from build123d import *

# Parameters (mm, degrees)
F0_R     = 2
F0_R_2   = 3
F0_R_3   = 1.5
F0_R_4   = 5
F1_DEPTH = 5
F2_R     = 1
F3_R     = 5
F4_DEPTH = 7
F6_W     = 20.916191861
F6_H     = 23.5347189009
F6_W_2   = 37.2305270284
F6_H_2   = 26.8968194723
F7_DEPTH = 25
F8_R     = 5


# Not quite as in the source:
# - a fillet or chamfer that OpenCascade refuses, or shapes differently, is made with other operations: its cross-section is extruded or revolved along the edge and cut away or added


with BuildPart() as f1:
    # F0 (on Top) → F1 (new body)
    with BuildSketch(Plane.XY):
        Polygon((-49.7560231508, 7), (-49.7560231508, 0), (76.2439768492, 0), (76.2439768492, 7), (33.2439768492, 7), (-6.7560231508, 7), align=None)
        with Locations((-45.7560231508, 3)):
            Circle(F0_R, mode=Mode.SUBTRACT)
        with Locations((72.2439768492, 3)):
            Circle(F0_R, mode=Mode.SUBTRACT)
        Polygon((-49.7560231508, 93.5), (-49.7560231508, 7), (-6.7560231508, 7), (-6.7560231508, 12), (33.2439768492, 12), (33.2439768492, 7), (76.2439768492, 7), (76.2439768492, 93.5), (33.2439768492, 93.5), (33.2439768492, 88.5), (-6.7560231508, 88.5), (-6.7560231508, 93.5), align=None)
        with Locations((-34.7560231508, 26.25)):
            Circle(F0_R_2, mode=Mode.SUBTRACT)
        with Locations((3.2439768492, 40.25)):
            Circle(F0_R_3, mode=Mode.SUBTRACT)
        with Locations((23.2439768492, 40.25)):
            Circle(F0_R_3, mode=Mode.SUBTRACT)
        with Locations((48.2439768492, 26.25)):
            Circle(F0_R_2, mode=Mode.SUBTRACT)
        with Locations((3.2439768492, 60.25)):
            Circle(F0_R_3, mode=Mode.SUBTRACT)
        with Locations((-34.7560231508, 74.25)):
            Circle(F0_R_2, mode=Mode.SUBTRACT)
        with Locations((13.2439768492, 50.25)):
            Circle(F0_R_4, mode=Mode.SUBTRACT)
        with Locations((23.2439768492, 60.25)):
            Circle(F0_R_3, mode=Mode.SUBTRACT)
        with Locations((48.2439768492, 74.25)):
            Circle(F0_R_2, mode=Mode.SUBTRACT)
        Polygon((-49.7560231508, 98.5), (-49.7560231508, 93.5), (-6.7560231508, 93.5), (33.2439768492, 93.5), (76.2439768492, 93.5), (76.2439768492, 98.5), align=None)
        with Locations((-34.7560231508, 26.25)):
            Circle(F0_R_2)
        with Locations((-34.7560231508, 26.25)):
            Circle(F0_R_3, mode=Mode.SUBTRACT)
        with Locations((-34.7560231508, 74.25)):
            Circle(F0_R_2)
        with Locations((-34.7560231508, 74.25)):
            Circle(F0_R_3, mode=Mode.SUBTRACT)
        with Locations((48.2439768492, 26.25)):
            Circle(F0_R_2)
        with Locations((48.2439768492, 26.25)):
            Circle(F0_R_3, mode=Mode.SUBTRACT)
        with Locations((48.2439768492, 74.25)):
            Circle(F0_R_2)
        with Locations((48.2439768492, 74.25)):
            Circle(F0_R_3, mode=Mode.SUBTRACT)
        with Locations((13.2439768492, 50.25)):
            Circle(F0_R_4)
        with Locations((3.2439768492, 60.25)):
            Circle(F0_R_3)
        with Locations((3.2439768492, 40.25)):
            Circle(F0_R_3)
        with Locations((23.2439768492, 40.25)):
            Circle(F0_R_3)
        with Locations((23.2439768492, 60.25)):
            Circle(F0_R_3)
    extrude(amount=F1_DEPTH)

    # F2
    f2_edges = [f1.edges().sort_by_distance(p)[0] for p in [
        (-6.756023, 12, 2.5),
        (33.243977, 12, 2.5),
        (-6.756023, 7, 2.5),
        (33.243977, 7, 2.5),
        (-6.756023, 88.5, 2.5),
        (-6.756023, 93.5, 2.5),
        (33.243977, 93.5, 2.5),
        (33.243977, 88.5, 2.5),
    ]]
    fillet(f2_edges, radius=F2_R)

    # F3
    f3_edges = [f1.edges().sort_by_distance(p)[0] for p in [
        (-49.756023, 0, 2.5),
        (76.243977, 0, 2.5),
        (76.243977, 98.5, 2.5),
        (-49.756023, 98.5, 2.5),
    ]]
    fillet(f3_edges, radius=F3_R)

    # F0 (on Top) → F4 (join)
    with BuildSketch(Plane.XY):
        with Locations((-34.7560231508, 74.25)):
            Circle(F0_R_2)
        with Locations((-34.7560231508, 74.25)):
            Circle(F0_R_3, mode=Mode.SUBTRACT)
        with Locations((-34.7560231508, 26.25)):
            Circle(F0_R_2)
        with Locations((-34.7560231508, 26.25)):
            Circle(F0_R_3, mode=Mode.SUBTRACT)
        with Locations((48.2439768492, 74.25)):
            Circle(F0_R_2)
        with Locations((48.2439768492, 74.25)):
            Circle(F0_R_3, mode=Mode.SUBTRACT)
        with Locations((48.2439768492, 26.25)):
            Circle(F0_R_2)
        with Locations((48.2439768492, 26.25)):
            Circle(F0_R_3, mode=Mode.SUBTRACT)
    extrude(amount=F4_DEPTH)

    # F5: fillet of radius 5 on 4 edges, made by hand

    # F5_s1 → F5_t2 (revolve)
    with BuildSketch(Plane.XZ.offset(-74.25)):
        with BuildLine():
            ThreePointArc((-27.7560231508, 5), (-29.9920911283, 5.527864045), (-31.7560231508, 7))
            Line((-31.7560231508, 7), (-31.7560231508, 5))
            Line((-31.7560231508, 5), (-27.7560231508, 5))
        make_face()
    revolve(axis=Axis((-34.7560231508, 74.25, 5), (0, 0, -1)))

    # F5_s3 → F5_t4 (revolve)
    with BuildSketch(Plane.XZ.offset(-26.25)):
        with BuildLine():
            ThreePointArc((-27.7560231508, 5), (-29.9920911283, 5.527864045), (-31.7560231508, 7))
            Line((-31.7560231508, 7), (-31.7560231508, 5))
            Line((-31.7560231508, 5), (-27.7560231508, 5))
        make_face()
    revolve(axis=Axis((-34.7560231508, 26.25, 5), (0, 0, -1)))

    # F5_s5 → F5_t6 (revolve)
    with BuildSketch(Plane.XZ.offset(-26.25)):
        with BuildLine():
            ThreePointArc((55.2439768492, 5), (53.0079088717, 5.527864045), (51.2439768492, 7))
            Line((51.2439768492, 7), (51.2439768492, 5))
            Line((51.2439768492, 5), (55.2439768492, 5))
        make_face()
    revolve(axis=Axis((48.2439768492, 26.25, 5), (0, 0, -1)))

    # F5_s7 → F5_t8 (revolve)
    with BuildSketch(Plane.XZ.offset(-74.25)):
        with BuildLine():
            ThreePointArc((51.2439768492, 7), (53.0079088717, 5.527864045), (55.2439768492, 5))
            Line((55.2439768492, 5), (51.2439768492, 5))
            Line((51.2439768492, 5), (51.2439768492, 7))
        make_face()
    revolve(axis=Axis((48.2439768492, 74.25, 5), (0, 0, -1)))

    # F6 (on face) → F7 (cut)
    with BuildSketch(Plane.XY.offset(5)):
        Polygon((31.9697726518, 84.2200964689), (-22.3512705415, 84.2200964689), (-22.3512705415, 62.1007867157), (-22.3512705415, 38.5660678148), (-22.3512705415, 16.3328051567), (31.9697726518, 16.3328051567), (31.9697726518, 37.4815165997), (31.9697726518, 64.378336072), align=None)
        with Locations((-32.8093664721, 50.3334272653)):
            Rectangle(F6_W, F6_H)
        with Locations((50.585036166, 50.9299263358)):
            Rectangle(F6_W_2, F6_H_2)
    extrude(amount=-F7_DEPTH, mode=Mode.SUBTRACT)

    # F8
    f8_edges = [f1.edges().sort_by_distance(p)[0] for p in [
        (-22.351271, 62.100787, 2.5),
        (31.969773, 64.378336, 2.5),
        (31.969773, 37.481517, 2.5),
        (-22.351271, 38.566068, 2.5),
        (-43.267462, 38.566068, 2.5),
        (-43.267462, 62.100787, 2.5),
        (-22.351271, 84.220096, 2.5),
        (31.969773, 84.220096, 2.5),
        (69.2003, 64.378336, 2.5),
        (69.2003, 37.481517, 2.5),
        (31.969773, 16.332805, 2.5),
        (-22.351271, 16.332805, 2.5),
    ]]
    fillet(f8_edges, radius=F8_R)


solid = f1.part
Input: part model. Units: mm. Frame: model coordinates. A direction names the side the tool comes from. Coordinates: 2 decimals unless noted, no trailing zeros. Loops run counter-clockwise (first coordinate to the right, second up) from the corner with the lowest first, then second, coordinate; pieces in that order, holes last. Notation, with made-up numbers: (24.5, 62.5) - (32.5, 62.5) arc R26 cw to (32.5, 98.5) - close; hole circle Ø1 at (74, 56). An arc over 180 degrees is marked (long way). Answer in a Markdown table with one row per item. Add a question column.
Item 1: Section query D-D on y = 26.25. Return the cut outline in (x, z), then the cut area to 3 significant figures.
Item 2: Section query A-A on x = 58.5. Return the cut outline in (y, z), then the cut area to 3 significant figures.
Item 3: Section query B-B on x = 20.5. Return the cut outline in (y, z).
Item 4: Access query for faces 4 (the cylindrical face through (-20.93, 17.84, 2.46)), 5 (the flat face through (14, 98.5, 2)). Directions: +Z, -Z, +X, -X, +Y, -Y. A direction counts if a zero-diameter tool reaches every point of the face in a straight line with its end or side. Return the directions, or none.
Item 5: Line query: line 1 along Y through (x, z) = (-6, 4); line 2 along X through (y, z) = (74.25, 4.75); line 3 along Y through (x, z) = (54.5, 1.25). Output: solid intervals per line, ascending. Write a range as [from, to].
Item 6: Mould query, pull axis X, two halves, no side actions, for faces 1 (the flat face through (14, 88.5, 2)), 2 (the flat face through (-34, 28, 7)), 3 (the flat face through (-49.756, 50, 2)). Classes: released by +X, released by -X, zero draft, split by the parting line, or undercut.
Item 7: Contact query for flat-ended pins moving along their axis: P1, Ø1.8, axis at x = 48.24, y = 74.25, coming from the +Z side; P2, Ø8, axis at x = -26, y = 38, coming from the -Z side; P3, Ø6.5, axis at x = -45.76, y = 3, coming from the +Z side. Output: stop coordinate, or through.
Item 8: Section query C-C on y = 3. Return the cut outline in (x, z), then the cut area to 3 significant figures.
Recorded:
| question | item | result |
|---|---|---|
| 1 | outline | (-49.76, 0) - (-36.26, 0) - (-36.26, 7) - (-37.76, 7) arc R5 cw to (-41.76, 5) - (-49.76, 5) - close; (-33.26, 0) - (-22.35, 0) - (-22.35, 5) - (-27.76, 5) arc R5 cw to (-31.76, 7) - (-33.26, 7) - close; (31.97, 0) - (46.74, 0) - (46.74, 7) - (45.24, 7) arc R5 cw to (41.24, 5) - (31.97, 5) - close; (49.74, 0) - (76.24, 0) - (76.24, 5) - (55.24, 5) arc R5 cw to (51.24, 7) - (49.74, 7) - close |
| 1 | area | 350 mm^2 |
| 2 | outline | (0, 0) - (37.48, 0) - (37.48, 5) - (0, 5) - close; (64.38, 0) - (98.5, 0) - (98.5, 5) - (64.38, 5) - close |
| 2 | area | 358 mm^2 |
| 3 | outline | (0, 0) - (7, 0) - (7, 5) - (0, 5) - close; (12, 0) - (16.33, 0) - (16.33, 5) - (12, 5) - close; (84.22, 0) - (88.5, 0) - (88.5, 5) - (84.22, 5) - close; (93.5, 0) - (98.5, 0) - (98.5, 5) - (93.5, 5) - close |
| 4 | face 4 | +Z, -Z |
| 4 | face 5 | +Z, -Z, +X, -X, +Y |
| 5 | line 1 | [0, 7.03], [11.97, 16.33], [84.22, 88.53], [93.47, 98.5] |
| 5 | line 2 | [-49.76, -36.26], [-33.26, -22.35], [31.97, 46.74], [49.74, 76.24] |
| 5 | line 3 | [0, 37.48], [64.38, 98.5] |
| 6 | face 1 | undercut |
| 6 | face 2 | zero draft |
| 6 | face 3 | released by -X |
| 7 | P1 | through |
| 7 | P2 | z = 0 |
| 7 | P3 | z = 5 |
| 8 | outline | (-49.34, 0) - (-47.76, 0) - (-47.76, 5) - (-49.34, 5) - close; (-43.76, 0) - (70.24, 0) - (70.24, 5) - (-43.76, 5) - close; (74.24, 0) - (75.83, 0) - (75.83, 5) - (74.24, 5) - close |
| 8 | area | 586 mm^2 |
